Input: part model. Units: mm. Frame: model coordinates. Face numbers are marked on the shaded views. A direction names the side the tool comes from. Round coordinates to 2 decimals unless told otherwise and drop trailing zeros. Loops run counter-clockwise (first coordinate to the right, second up) from the corner with the lowest first, then second, coordinate; pieces in that order, holes last. Notation, with made-up numbers: (-9.5, 32.5) -> (-1.5, 32.5) arc R29 cw to (-1.5, 58.5) -> close; hole circle Ø6 at (73, 27). An arc over 180 degrees is marked (long way). One line per question, with ' | ' between items. Start each with the question number.
Q1. Cut plane C-C on x = 4.5. Return loops of the section in (y, z).
Q2. Cut plane B-B on z = 20. Return loops of the section in (x, y), and give its area (3 significant figures).
Q3. Material intervals for L1, parallel to Z at x = 5.5, y = -6; L2, parallel to X at y = -4.5, z = 4; L3, parallel to Z at x = -8.5, y = -10, sorted ascending.
Q4. Cut plane A-A on x = -9. Return loops of the section in (y, z), and give its area (3 significant figures).
Q5. Mould query, pull axis Z, two halves, no side actions, for the marked faces 4, 5 and 6. Classes: pulls with the +Z half, pulls with the -Z half, needs draft (parallel to the pull), parting line crosses it, or undercut.
Q6. Contact query for flat-ended pins moving along their axis: P1, Ø6, axis at y = 6.5, z = 33.5, coming from the +X side; P2, Ø6, axis at x = -1.5, z = 7, coming from the -Y side; P3, Ø6, axis at y = -4.5, z = 28.5, coming from the +X side. Output: stop coordinate, or through.
Q7. Access query for the marked faces 1, 2 and 3. Directions: +Z, -Z, +X, -X, +Y, -Y. A direction counts if a zero-diameter tool reaches every point of the face in a straight line with its end or side. Return the directions, or none.
from build123d import *

# Parameters (mm, degrees)
SKETCH1_W           = 19.5
SKETCH1_H           = 32.5
BOSS_EXTRUDE1_DEPTH = 26
SKETCH2_R           = 6
BOSS_EXTRUDE2_DEPTH = 9
BOSS_EXTRUDE3_START = -2
BOSS_EXTRUDE3_DEPTH = 0.5
SWEEP1_OUTLINE_W    = 2.5
SWEEP1_OUTLINE_H    = 18.679041634
FILLET1_R           = 1.5


# Read off the part's stored shape, not the designer's step: Sweep1
with BuildPart() as part:
    # Sketch1 → Boss-Extrude1 (new body)
    with BuildSketch(Plane.XY):
        Rectangle(SKETCH1_W, SKETCH1_H)
    extrude(amount=BOSS_EXTRUDE1_DEPTH)

    # Sketch2 → Boss-Extrude2 (add)
    with BuildSketch(Plane.XY.offset(26)):
        with Locations(Location((0, 0, 0), (0, 0, 180))):
            Circle(SKETCH2_R)
    extrude(amount=BOSS_EXTRUDE2_DEPTH)

    # Sketch3 → Boss-Extrude3 (add)
    with BuildSketch(Plane.XY.offset(35).offset(BOSS_EXTRUDE3_START)):
        with BuildLine():
            Line((8, 9.276987658), (8, 17))
            Line((8, 17), (-8, 17))
            Line((-8, 17), (-8, 9.276987658))
            ThreePointArc((-8, 9.276987658), (-12.25, 0), (-8, -9.276987658))
            Line((-8, -9.276987658), (-8, -17))
            Line((-8, -17), (8, -17))
            Line((8, -17), (8, -9.276987658))
            ThreePointArc((8, -9.276987658), (12.25, 0), (8, 9.276987658))
        make_face()
    extrude(amount=-BOSS_EXTRUDE3_DEPTH)

    # Sweep1 outline → Sweep1 (revolve)
    with BuildSketch(Plane(origin=(0, 8.75, 2.344555434), x_dir=(1, 0, 0), z_dir=(0, 0.965925826289068, 0.258819045102522))):
        with Locations((1.25, -42.467883103)):
            Rectangle(SWEEP1_OUTLINE_W, SWEEP1_OUTLINE_H)
    revolve(axis=Axis((0, 8.75, 2.344555434), (0, 0.258819045102522, -0.965925826289068)))

    # Fillet1
    fillet1_edges = [part.edges().sort_by_distance(p)[0] for p in [
        (-2.5, -4.658742812, 52.386664873),
    ]]
    fillet(fillet1_edges, radius=FILLET1_R)


solid = part.part
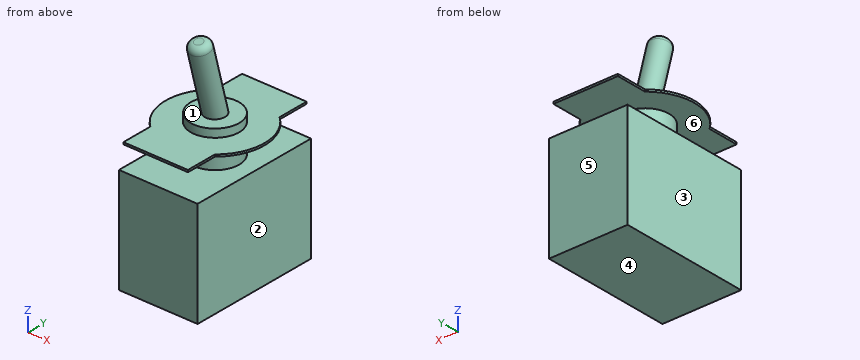
Results:
1) outline: (-17, 32.5) -> (-3.97, 32.5) -> (-3.97, 26) -> (-16.25, 26) -> (-16.25, 0) -> (16.25, 0) -> (16.25, 26) -> (3.97, 26) -> (3.97, 32.5) -> (17, 32.5) -> (17, 33) -> (3.97, 33) -> (3.97, 35) -> (-3.97, 35) -> (-3.97, 33) -> (-17, 33) -> close
2) outline: (-9.75, -16.25) -> (9.75, -16.25) -> (9.75, 16.25) -> (-9.75, 16.25) -> close | area: 634 mm^2
3) L1: 0 to 26, 32.5 to 33 | L2: -9.75 to 9.75 | L3: 0 to 26
4) outline: (-16.25, 0) -> (16.25, 0) -> (16.25, 26) -> (-16.25, 26) -> close; (-8.31, 32.5) -> (8.31, 32.5) -> (8.31, 33) -> (-8.31, 33) -> close | area: 853 mm^2
5) face 4: pulls with the -Z half | face 5: needs draft | face 6: undercut
6) P1: x = 11.73 | P2: y = -16.25 | P3: x = 9.75
7) face 1: none | face 2: -Z, +X, +Y, -Y | face 3: -Z, -X, +Y, -Y
